```python
from build123d import *

# Parameters (mm, degrees)
F0_W     = 71
F0_H     = 58
F1_DEPTH = 5.00012
F2_R     = 3
F3_R     = 1.651
F4_DEPTH = 5.00112
F5_R     = 3.556
F5_R_2   = 1.778
F6_DEPTH = 2.5
F8_DEPTH = 3.5


# Not quite as in the source:
# - after a boolean that leaves OpenCascade's solid faulty, fix() repairs it
# - a feature names something its author has since deleted; it is built from what else it names


with BuildPart() as f1:
    # F0 (on Top) → F1 (new body)
    with BuildSketch(Plane.XY):
        Rectangle(F0_W, F0_H)
    extrude(amount=F1_DEPTH)

    # F2
    f2_edges = [f1.edges().sort_by_distance(p)[0] for p in [
        (-35.5, 29, 2.50006),
        (35.5, 29, 2.50006),
        (35.5, -29, 2.50006),
        (-35.5, -29, 2.50006),
    ]]
    fillet(f2_edges, radius=F2_R)

    # F3 (on face) → F4 (cut, through all)
    with BuildSketch(Plane.XY.offset(5.00012)):
        with Locations((-31.1785, 24.6761)):
            Circle(F3_R)
        with Locations((-31.1785, -24.6761)):
            Circle(F3_R)
        with Locations((31.1785, -24.6761)):
            Circle(F3_R)
        with Locations((31.1785, 24.6761)):
            Circle(F3_R)
    extrude(amount=-F4_DEPTH, mode=Mode.SUBTRACT)

    # F5 (on face) → F6 (join)
    with BuildSketch(Plane(origin=(0, 0, 0), x_dir=(1, 0, 0), z_dir=(0, 0, -1))):
        with Locations((-28, 17.875)):
            Circle(F5_R)
        with Locations((-28, 17.875)):
            Circle(F5_R_2, mode=Mode.SUBTRACT)
        with Locations((28, 17.875)):
            Circle(F5_R)
        with Locations((28, 17.875)):
            Circle(F5_R_2, mode=Mode.SUBTRACT)
        with Locations((28, -17.875)):
            Circle(F5_R)
        with Locations((28, -17.875)):
            Circle(F5_R_2, mode=Mode.SUBTRACT)
        with Locations((-28, -17.875)):
            Circle(F5_R)
        with Locations((-28, -17.875)):
            Circle(F5_R_2, mode=Mode.SUBTRACT)
    extrude(amount=F6_DEPTH)

    # F7 (on face) → F8 (cut)
    with BuildSketch(Plane(origin=(0, 0, 0), x_dir=(1, 0, 0), z_dir=(0, 0, -1))):
        with BuildLine():
            ThreePointArc((28, 14.319), (25.4855282861, 15.3605282861), (24.444, 17.875))
            Line((24.444, 17.875), (-24.444, 17.875))
            ThreePointArc((-24.444, 17.875), (-25.4855282861, 15.3605282861), (-28, 14.319))
            Line((-28, 14.319), (-28, -14.319))
            ThreePointArc((-28, -14.319), (-25.4855282861, -15.3605282861), (-24.444, -17.875))
            Line((-24.444, -17.875), (24.444, -17.875))
            ThreePointArc((24.444, -17.875), (25.4855282861, -15.3605282861), (28, -14.319))
            Line((28, -14.319), (28, 14.319))
        make_face()
    extrude(amount=-F8_DEPTH, mode=Mode.SUBTRACT)

    add(f1.part.fix(), mode=Mode.REPLACE)


solid = f1.part
```
Design review of the part built by this model. Coordinates are the model's own, in mm. A direction names the side the tool comes from. Give positions to 0.01 mm unless a question says otherwise; leave off trailing zeros. Write each loop counter-clockwise with the first axis right and the second up, starting at its lowest first coordinate (ties: lowest second). Pieces come first, ordered by that corner, then holes. Notation, with made-up numbers: (37.25, 45) - (81.25, 45) arc R28 cw to (81.25, 71) - close; hole circle Ø6 at (-30, -38). An arc over 180 degrees is marked (long way). Return JSON: item names as keys, results as strings. Group by question number.
(1) We need section A-A, the plane x = 8. Give the boundary of the cut face in (y, z) (3 decimals), then the cut area to 3 significant figures.
(2) Machinability: for faces 4 (the flat face through (0, 0, 5)), 5 (the cylindrical face through (26.224, 17.797, -1.232)), which of the approach directions +Z, -Z, +X, -X, +Y, -Y give a long, thin tool a straight path to every point of the face, cutting with its end or side? Answer none if there is none.
(3) Insertion check: pin 1 (1.1 mm diameter, centred on x = 27, y = -17.5, fed in from -Z); pin 2 (2.5 mm diameter, centred on x = 31.18, y = -24.68, fed in from -Z); pin 3 (5 mm diameter, centred on x = -23, y = 6.5, fed in from -Z). Each pin has a flat end and moves straight along its axis. Give the tip position at first contact, or say it passes through.
(4) We need section C-C, the plane z = 2.25. Give the boundary of the cut face in (x, y) (1 decimal), then the cut area to 3 significant figures.
(5) To check wall thickness, follow probe 1 along Y at (x, z) = (-28, -1.45); probe 2 along X at (y, z) = (-24, 3.25); probe 3 along X at (y, z) = (9, 0.25). State the ranges of each line that lie inside material, in increasing order.
(6) We need section B-B, the plane y = 13. Give the boundary of the cut face in (x, z).
(7) Mouldability with a two-part tool opening along X and no side actions: class faces 1 (the flat face through (0, 17.875, 2)), 2 (the cylindrical face through (34.64, 28.1, 2.54)), 3 (the flat face through (26, -17, -2.5)) as +X half, -X half, draft (parallel to the pull), parting line (faces both ways), or undercut.
Reported:
{
 "1": {"outline": "(-29, 0) - (-17.875, 0) - (-17.875, 3.5) - (17.875, 3.5) - (17.875, 0) - (29, 0) - (29, 5) - (-29, 5) - close", "area": "165 mm2"},
 "2": {"face 4": "+Z, +X, -X, +Y, -Y", "face 5": "-Z"},
 "3": {"pin 1": "stops at z = 0", "pin 2": "passes through", "pin 3": "stops at z = 3.5"},
 "4": {"outline": "(-35.5, -26) arc R3 ccw to (-32.5, -29) - (32.5, -29) arc R3 ccw to (35.5, -26) - (35.5, 26) arc R3 ccw to (32.5, 29) - (-32.5, 29) arc R3 ccw to (-35.5, 26) - close; hole circle Ø3.3 at (-31.2, -24.7); hole circle Ø3.3 at (-31.2, 24.7); hole (-28, -14.3) arc R3.6 cw to (-24.4, -17.9) - (24.4, -17.9) arc R3.6 cw to (28, -14.3) - (28, 14.3) arc R3.6 cw to (24.4, 17.9) - (-24.4, 17.9) arc R3.6 cw to (-28, 14.3) - close; hole circle Ø3.3 at (31.2, -24.7); hole circle Ø3.3 at (31.2, 24.7)", "area": "2,110 mm2"},
 "5": {"probe 1": "y = -21.43 to -19.65, -16.1 to -14.32, 14.32 to 16.1, 19.65 to 21.43", "probe 2": "x = -35.5 to -32.68, -29.67 to 29.67, 32.68 to 35.5", "probe 3": "x = -35.5 to -28, 28 to 35.5"},
 "6": {"outline": "(-35.5, 0) - (-28, 0) - (-28, 3.5) - (28, 3.5) - (28, 0) - (35.5, 0) - (35.5, 5) - (-35.5, 5) - close"},
 "7": {"face 1": "undercut", "face 2": "+X half", "face 3": "draft"}
}
